```python
from build123d import *

# Parameters (mm, degrees)
SKETCH070_R       = 6
PAD046_DEPTH      = 10
SKETCH071_R       = 10
PAD047_DEPTH      = 2
SKETCH072_R       = 9.25
PAD048_DEPTH      = 3
SKETCH073_R       = 8.875
POCKET068_DEPTH   = 0.2
POCKET068_FACE9_R = 8.875
PAD049_DEPTH      = 3.2


with BuildPart() as part:
    # Sketch070 → Pad046 (new body)
    with BuildSketch(Plane.XY):
        Circle(SKETCH070_R)
    extrude(amount=PAD046_DEPTH)

    # Sketch071 (on Face3 of Pad046) → Pad047 (join)
    with BuildSketch(Plane.XY.offset(10)):
        Circle(SKETCH071_R)
    extrude(amount=PAD047_DEPTH)

    # Sketch072 (on Face3 of Pad047) → Pad048 (join)
    with BuildSketch(Plane.XY.offset(12)):
        Circle(SKETCH072_R)
    extrude(amount=PAD048_DEPTH)

    # Sketch073 (on Face7 of Pad048) → Pocket068 (cut)
    with BuildSketch(Plane.XY.offset(15)):
        Circle(SKETCH073_R)
    extrude(amount=-POCKET068_DEPTH, mode=Mode.SUBTRACT)

    # Pocket068 Face9 → Pad049 (add)
    with BuildSketch(Plane(origin=(0, 0, 14.8), x_dir=(0, 1, 0), z_dir=(0, 0, 1))):
        Circle(POCKET068_FACE9_R)
    extrude(amount=PAD049_DEPTH)

    # Sketch074 → Groove (revolve, cut)
    with BuildSketch(Plane.XZ):
        with BuildLine():
            ThreePointArc((8.875, 15), (4.684658, 17.231174), (0, 18))
            Line((0, 19), (0, 18))
            Line((0, 19), (8.875, 19))
            Line((8.875, 19), (8.875, 15))
        make_face()
    revolve(axis=Axis((0, 0, 0), (0, 0, 1)), mode=Mode.SUBTRACT)


with BuildPart() as part_1:
    # Body006 placement: moved
    add(part.part.moved(Location((-0.09, 20.45, -3.6))))


solid = part_1.part
```
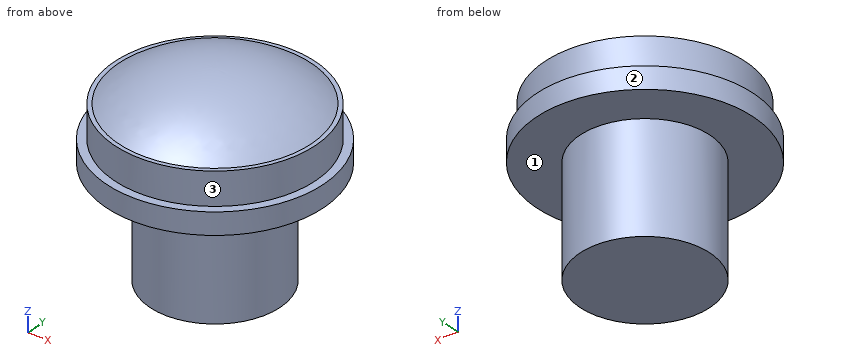
The listing builds one solid part. Answer for the finished solid, in the listing's coordinates (mm). Face numbers are marked on the shaded views. A direction names the side the tool comes from. Coordinates: 2 decimals unless noted, no trailing zeros. Loops run counter-clockwise (first coordinate to the right, second up) from the corner with the lowest first, then second, coordinate; pieces in that order, holes last. Notation, with made-up numbers: (63.5, -11.75) - (95.5, -11.75) arc R6 ccw to (95.5, -5.75) - close; hole circle Ø11 at (89, 52). An arc over 180 degrees is marked (long way). Use a Markdown table: item, result. Add a question column.
1) For the marked faces 1, 2 and 3, determine the directions among +Z, -Z, +X, -X, +Y, -Y from which every point of the face is accessible in a straight line to the end or side of a thin tool.
2) The part is cut by section A-A, the plane z = 4.5. Give the vertices of the cut face in (x, y).
3) Find the intervals of material crossed by line 1 (Z direction, x = -5, y = 29); line 2 (Z direction, x = -7, y = 14.75); line 3 (Y direction, x = 2.75, z = 4), in increasing order.
4) Given pin 1 (5 mm diameter, centred on y = 13, z = 10.5, fed in from -X); pin 2 (3 mm diameter, centred on y = 24.5, z = 1, fed in from +X); pin 3 (4 mm diameter, centred on x = -7.5, z = -1.5, fed in from +Y); pin 4 (10 mm diameter, centred on x = -0.5, y = 16.5, fed in from +Z), each flat-ended and moving along its own axis, determine where each tip first touches the part or whether it passes through.
Here are the results:
| question | item | result |
|---|---|---|
| 1 | face 1 | -Z |
| 1 | face 2 | +Z, -Z |
| 1 | face 3 | +Z |
| 2 | outline | circle Ø12 at (-0.09, 20.45) |
| 3 | line 1 | z = 6.4 to 8.4 |
| 3 | line 2 | z = 6.4 to 11.4 |
| 3 | line 3 | y = 15.16 to 25.74 |
| 4 | pin 1 | stops at x = -8.02 |
| 4 | pin 2 | stops at x = 5.34 |
| 4 | pin 3 | stops at y = 23.04 |
| 4 | pin 4 | stops at z = 14.4 |
